from build123d import *

# Parameters (mm, degrees)
ESQUISSE2_W                  = 165
ESQUISSE2_H                  = 165
BASE_DEPTH                   = 30
ESQUISSE3_R                  = 15
BLOC_MOTEUR_1_DEPTH          = 80
ESQUISSE4_W                  = 10
ESQUISSE4_H                  = 22.360679774
ACCES_MOTEUR_DEPTH           = 37
ESQUISSE6_R                  = 16.01
BLOC_MOTEUR_2_DEPTH          = 37
ESQUISSE7_R                  = 2.5
VIS_MOTEUR_DEPTH             = 121.467838032
ESQUISSE8_R                  = 2.5
VIS_PATIN_DEPTH              = 121.467838032
ESQUISSE12_R                 = 30
ESPACE_ROUE_DEPTH            = 10
ESQUISSE23_W                 = 10
ESQUISSE23_H                 = 30
VIDE_TIGE_DEPTH              = 10
VIDE_VIS_REACH               = 180.133
ESQUISSE25_R                 = 2.5
ENL_V_MAT_EXTRU_1_DEPTH      = 10
ENL_V_MAT_EXTRU_1_DEPTH_BACK = 10
BOSS_EXTRU_1_DEPTH           = 2.5
BOSS_EXTRU_1_DEPTH_BACK      = 2.5


with BuildPart() as part:
    # Esquisse2 → BASE (new body)
    with BuildSketch(Plane(origin=(0, 0, 0), x_dir=(1, 0, 0), z_dir=(0, 1, 0))):
        Rectangle(ESQUISSE2_W, ESQUISSE2_H)
    extrude(amount=BASE_DEPTH)

    # Esquisse3 → BLOC MOTEUR 1. (cut)
    with BuildSketch(Plane(origin=(82.5, 0, 0), x_dir=(0, 0, -1), z_dir=(1, 0, 0))):
        with Locations((50, 10)):
            Circle(ESQUISSE3_R)
    bloc_moteur_1 = extrude(amount=-BLOC_MOTEUR_1_DEPTH, mode=Mode.SUBTRACT)

    # Esquisse4 → ACCES MOTEUR (cut)
    with BuildSketch(Plane.XZ):
        with Locations((7.5, -50)):
            Rectangle(ESQUISSE4_W, ESQUISSE4_H)
    acces_moteur = extrude(amount=-ACCES_MOTEUR_DEPTH, mode=Mode.SUBTRACT)

    # Esquisse6 → BLOC MOTEUR 2 (cut)
    with BuildSketch(Plane(origin=(82.5, 0, 0), x_dir=(0, 0, -1), z_dir=(1, 0, 0))):
        with Locations((50, 10)):
            Circle(ESQUISSE6_R)
    bloc_moteur_2 = extrude(amount=-BLOC_MOTEUR_2_DEPTH, mode=Mode.SUBTRACT)

    # SYM BLOC MOTEUR: BLOC MOTEUR 1., ACCES MOTEUR, BLOC MOTEUR 2 across plane
    add(bloc_moteur_1.mirror(Plane(origin=(0, 0, 0), x_dir=(0, 0, 1), z_dir=(1, 0, 0))), mode=Mode.SUBTRACT)
    add(acces_moteur.mirror(Plane(origin=(0, 0, 0), x_dir=(0, 0, 1), z_dir=(1, 0, 0))), mode=Mode.SUBTRACT)
    add(bloc_moteur_2.mirror(Plane(origin=(0, 0, 0), x_dir=(0, 0, 1), z_dir=(1, 0, 0))), mode=Mode.SUBTRACT)

    # Esquisse7 → VIS MOTEUR (cut, through all)
    with BuildSketch(Plane.XZ):
        with Locations(Location((-64, -27.497196314, 0), (0, 0, 270))):
            Circle(ESQUISSE7_R)
        with Locations(Location((-24, -28.819660113, 0), (0, 0, 270))):
            Circle(ESQUISSE7_R)
        with Locations(Location((-24, -71.180339887, 0), (0, 0, 270))):
            Circle(ESQUISSE7_R)
        with Locations(Location((-64, -72.502803686, 0), (0, 0, 270))):
            Circle(ESQUISSE7_R)
    vis_moteur = extrude(amount=-VIS_MOTEUR_DEPTH, mode=Mode.SUBTRACT)

    # SYM VIS: VIS MOTEUR across plane
    add(vis_moteur.mirror(Plane(origin=(0, 0, 0), x_dir=(0, 0, 1), z_dir=(1, 0, 0))), mode=Mode.SUBTRACT)

    # Esquisse8 → VIS PATIN (cut, through all)
    with BuildSketch(Plane.XZ):
        with Locations(Location((-52.5, 52.5, 0), (0, 0, 270))):
            Circle(ESQUISSE8_R)
        with Locations(Location((52.5, 52.5, 0), (0, 0, 270))):
            Circle(ESQUISSE8_R)
    extrude(amount=-VIS_PATIN_DEPTH, mode=Mode.SUBTRACT)

    # Esquisse12 → ESPACE ROUE (cut)
    with BuildSketch(Plane.ZY.offset(82.5)):
        with Locations((-50, 10)):
            Circle(ESQUISSE12_R)
    espace_roue = extrude(amount=-ESPACE_ROUE_DEPTH, mode=Mode.SUBTRACT)

    # SYM ESPACE ROUE: ESPACE ROUE across plane
    add(espace_roue.mirror(Plane(origin=(0, 0, 0), x_dir=(0, 0, 1), z_dir=(1, 0, 0))), mode=Mode.SUBTRACT)

    # Esquisse23 → VIDE TIGE (cut)
    with BuildSketch(Plane(origin=(82.5, 0, 0), x_dir=(0, 0, -1), z_dir=(1, 0, 0))):
        with Locations((-72.5, 15)):
            Rectangle(ESQUISSE23_W, ESQUISSE23_H)
        with Locations((7.5, 15)):
            Rectangle(ESQUISSE23_W, ESQUISSE23_H)
    vide_tige = extrude(amount=-VIDE_TIGE_DEPTH, mode=Mode.SUBTRACT)

    # SYM TIGE: VIDE TIGE across plane
    add(vide_tige.mirror(Plane(origin=(0, 0, 0), x_dir=(0, 0, 1), z_dir=(1, 0, 0))), mode=Mode.SUBTRACT)

    # Esquisse25 → VIDE VIS (cut, up to next)
    with BuildSketch(Plane(origin=(72.5, 0, 0), x_dir=(0, 0, -1), z_dir=(1, 0, 0)), mode=Mode.PRIVATE) as vide_vis_sk1:
        with Locations((-72.5, 25)):
            Circle(ESQUISSE25_R)
    vide_vis_tool1 = extrude(vide_vis_sk1.sketch, amount=-VIDE_VIS_REACH, mode=Mode.PRIVATE) & part.part
    # Esquisse25 → VIDE VIS (cut, up to next)
    with BuildSketch(Plane(origin=(72.5, 0, 0), x_dir=(0, 0, -1), z_dir=(1, 0, 0)), mode=Mode.PRIVATE) as vide_vis_sk2:
        with Locations((-72.5, 15)):
            Circle(ESQUISSE25_R)
    vide_vis_tool2 = extrude(vide_vis_sk2.sketch, amount=-VIDE_VIS_REACH, mode=Mode.PRIVATE) & part.part
    # Esquisse25 → VIDE VIS (cut, up to next)
    with BuildSketch(Plane(origin=(72.5, 0, 0), x_dir=(0, 0, -1), z_dir=(1, 0, 0)), mode=Mode.PRIVATE) as vide_vis_sk3:
        with Locations((-72.5, 5)):
            Circle(ESQUISSE25_R)
    vide_vis_tool3 = extrude(vide_vis_sk3.sketch, amount=-VIDE_VIS_REACH, mode=Mode.PRIVATE) & part.part
    # Esquisse25 → VIDE VIS (cut, up to next)
    with BuildSketch(Plane(origin=(72.5, 0, 0), x_dir=(0, 0, -1), z_dir=(1, 0, 0)), mode=Mode.PRIVATE) as vide_vis_sk4:
        with Locations(Location((7.5, 5, 0), (0, 0, 180))):
            Circle(ESQUISSE25_R)
    vide_vis_tool4 = extrude(vide_vis_sk4.sketch, amount=-VIDE_VIS_REACH, mode=Mode.PRIVATE) & part.part
    # Esquisse25 → VIDE VIS (cut, up to next)
    with BuildSketch(Plane(origin=(72.5, 0, 0), x_dir=(0, 0, -1), z_dir=(1, 0, 0)), mode=Mode.PRIVATE) as vide_vis_sk5:
        with Locations(Location((7.5, 25, 0), (0, 0, 180))):
            Circle(ESQUISSE25_R)
    vide_vis_tool5 = extrude(vide_vis_sk5.sketch, amount=-VIDE_VIS_REACH, mode=Mode.PRIVATE) & part.part
    # Esquisse25 → VIDE VIS (cut, up to next)
    with BuildSketch(Plane(origin=(72.5, 0, 0), x_dir=(0, 0, -1), z_dir=(1, 0, 0)), mode=Mode.PRIVATE) as vide_vis_sk6:
        with Locations(Location((7.5, 15, 0), (0, 0, 180))):
            Circle(ESQUISSE25_R)
    vide_vis_tool6 = extrude(vide_vis_sk6.sketch, amount=-VIDE_VIS_REACH, mode=Mode.PRIVATE) & part.part
    add(vide_vis_tool1.solids().sort_by_distance((72.5, 25, 72.5))[0], mode=Mode.SUBTRACT)
    add(vide_vis_tool2.solids().sort_by_distance((72.5, 15, 72.5))[0], mode=Mode.SUBTRACT)
    add(vide_vis_tool3.solids().sort_by_distance((72.5, 5, 72.5))[0], mode=Mode.SUBTRACT)
    add(vide_vis_tool4.solids().sort_by_distance((72.5, 5, -7.5))[0], mode=Mode.SUBTRACT)
    add(vide_vis_tool5.solids().sort_by_distance((72.5, 25, -7.5))[0], mode=Mode.SUBTRACT)
    add(vide_vis_tool6.solids().sort_by_distance((72.5, 15, -7.5))[0], mode=Mode.SUBTRACT)

    # Esquisse27 → Enlèv. mat.-Extru.1 (cut, two sides: drawn at the far end of the back side and taken through both)
    with BuildSketch(Plane(origin=(0, 15, 0), x_dir=(1, 0, 0), z_dir=(0, 1, 0)).offset(-ENL_V_MAT_EXTRU_1_DEPTH_BACK)):
        Polygon((-77.5, -62.5), (-77.5, -2.5), (-68.5, -2.5), (-68.5, 16.142194012), (-68.5, 33.497196314), (-45.5, 33.497196314), (-45.5, 34.819660113), (45.5, 34.819660113), (45.5, 33.497196314), (68.5, 33.497196314), (68.5, 16.142194012), (68.5, -2.5), (77.5, -2.5), (77.5, -62.5), (67.5, -62.5), (67.5, -77.5), (-67.5, -77.5), (-67.5, -62.5), align=None)
        Polygon((-68.5, 66.502803686), (-45.5, 66.502803686), (-45.5, 65.180339887), (45.5, 65.180339887), (45.5, 66.502803686), (68.5, 66.502803686), (68.5, 77.5), (-68.5, 77.5), align=None)
    extrude(amount=ENL_V_MAT_EXTRU_1_DEPTH + ENL_V_MAT_EXTRU_1_DEPTH_BACK, mode=Mode.SUBTRACT)

    # Esquisse29 → Boss.-Extru.1 (add, two sides: drawn at the far end of the back side and taken through both)
    with BuildSketch(Plane(origin=(0, 15, 0), x_dir=(1, 0, 0), z_dir=(0, 1, 0)).offset(-BOSS_EXTRU_1_DEPTH_BACK)):
        with BuildLine():
            Line((-76.098768454, 2.5), (0, -29.784326011))
            Line((0, -29.784326011), (76.098768454, 2.5))
            Line((76.098768454, 2.5), (82.5, 2.5))
            Line((82.5, 2.5), (82.5, -0.215673989))
            Line((82.5, -0.215673989), (6.401231546, -32.5))
            Line((6.401231546, -32.5), (50.38861991, -51.161316275))
            ThreePointArc((50.38861991, -51.161316275), (51.523625383, -54.801454455), (54.929888079, -53.087914893))
            Line((54.929888079, -53.087914893), (82.5, -64.784326011))
            Line((82.5, -64.784326011), (82.5, -67.5))
            Line((82.5, -67.5), (76.098768454, -67.5))
            Line((76.098768454, -67.5), (0, -35.215673989))
            Line((0, -35.215673989), (-76.098768454, -67.5))
            Line((-76.098768454, -67.5), (-82.5, -67.5))
            Line((-82.5, -67.5), (-82.5, -64.784326011))
            Line((-82.5, -64.784326011), (-54.929888079, -53.087914893))
            ThreePointArc((-54.929888079, -53.087914893), (-51.523625383, -54.801454455), (-50.38861991, -51.161316275))
            Line((-50.38861991, -51.161316275), (-6.401231546, -32.5))
            Line((-6.401231546, -32.5), (-82.5, -0.215673989))
            Line((-82.5, -0.215673989), (-82.5, 2.5))
            Line((-82.5, 2.5), (-76.098768454, 2.5))
        make_face()
    extrude(amount=BOSS_EXTRU_1_DEPTH + BOSS_EXTRU_1_DEPTH_BACK)


solid = part.part
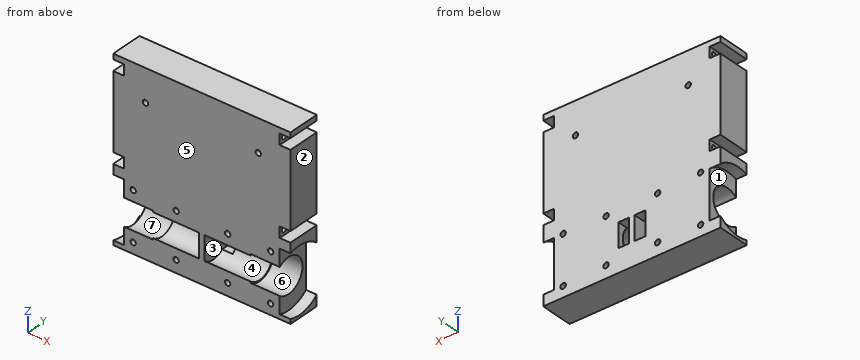
Input: part model. Units: mm. Frame: model coordinates. Face numbers are marked on the shaded views. A direction names the side the tool comes from. Give positions to 0.01 mm unless a question says otherwise; leave off trailing zeros. Order: outer loops, then holes, each group sorted by start corner. A loop starts at its lowest first (then second) coordinate and runs counter-clockwise, first axis right, second up. Notation, with made-up numbers: (-20, -37.5) - (34, -37.5) arc R23 ccw to (34, -12.5) - close; hole circle Ø3 at (-18, -16.75). An arc over 180 degrees is marked (long way). Answer as a JSON object with one key per item and string values. Group by question number.
Q1. Mould query, pull axis X, two halves, no side actions, for the marked faces 1, 2, 3 and 4. Classes: pulls with the +X half, pulls with the -X half, needs draft (parallel to the pull), parting line crosses it, or undercut.
Q2. Cut plane A-A, the plane z = 45.5. Output: boundary loops of the cut face in (x, y).
Q3. First-contact query: pin 1 Ø4 at (x, z) = (-64, -27.5) entering from -Y; pin 2 Ø8 at (y, z) = (14, -7.5) entering from +X. Flat tips, straight axial feed; report the tip coordinate or a pass-through.
Q4. Line query: probe 1 along X at (y, z) = (27, -57); probe 2 along Y at (x, z) = (68, 0); probe 3 along X at (y, z) = (11.5, -32). Output: solid intervals per line, ascending.
Q5. Cut plane B-B, the plane y = 10. Count the separate pieces of the cut face and the enclosed holes in it, then the cut area to 3 significant figures.
Q6. Set-up query: the marked faces 5, 6 and 7. Return all of +Z, -Z, +X, -X, +Y, -Y with unobstructed straight access to the full face (end or side cutting, diameter ignored); none if empty.
Results:
{
 "1": {"face 1": "pulls with the -X half", "face 2": "pulls with the +X half", "face 3": "undercut", "face 4": "needs draft"},
 "2": {"outline": "(-82.5, 0) - (82.5, 0) - (82.5, 30) - (-82.5, 30) - close; (-37.04, 12.5) - (-24.24, 12.5) - (-24.24, 17.5) - (-37.04, 17.5) - close; (24.24, 12.5) - (37.04, 12.5) - (37.04, 17.5) - (24.24, 17.5) - close; hole (-77.5, 5) - (77.5, 5) - (77.5, 25) - (-77.5, 25) - close"},
 "3": {"pin 1": "through", "pin 2": "x = 72.5"},
 "4": {"probe 1": "-72.5 to -12.5, -2.5 to 2.5, 12.5 to 72.5", "probe 2": "0 to 5, 25 to 30", "probe 3": "-72.5 to -68.5, 68.5 to 72.5"},
 "5": {"separate pieces": "3", "enclosed holes": "0", "area": "3,310 mm^2"},
 "6": {"face 5": "+Z, -Z, +X, -X, -Y", "face 6": "+X", "face 7": "-X"}
}
